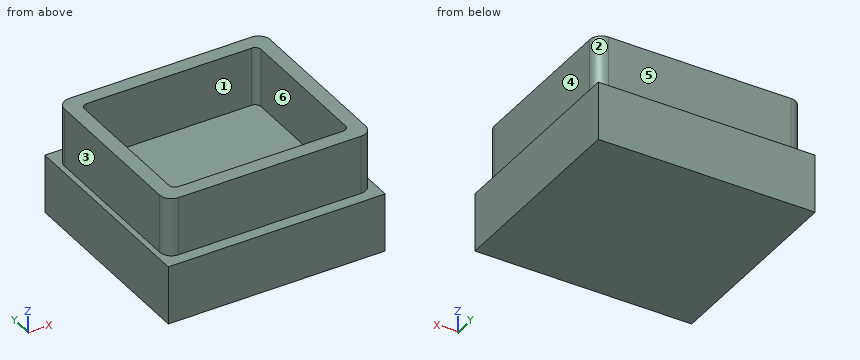
```python
from build123d import *

# Parameters (mm, degrees)
F0_W     = 89.387954
F0_H     = 77.989534
F0_W_2   = 76.687954
F0_H_2   = 65.289534
F1_DEPTH = 25.4
F2_R     = 5.08
F3_R     = 2.54
F4_W     = 94.174876
F4_H     = 87.917894
F5_DEPTH = 25.4


with BuildPart() as f1:
    # F0 (on Top) → F1 (new body)
    with BuildSketch(Plane.XY):
        Rectangle(F0_W, F0_H)
        Rectangle(F0_W_2, F0_H_2, mode=Mode.SUBTRACT)
    extrude(amount=F1_DEPTH)

    # F2
    f2_edges = [f1.edges().sort_by_distance(p)[0] for p in [
        (-44.693977, -38.994767, 12.7),
        (44.693977, -38.994767, 12.7),
        (44.693977, 38.994767, 12.7),
        (-44.693977, 38.994767, 12.7),
    ]]
    fillet(f2_edges, radius=F2_R)

    # F3
    f3_edges = [f1.edges().sort_by_distance(p)[0] for p in [
        (-38.343977, 32.644767, 12.7),
        (38.343977, 32.644767, 12.7),
        (38.343977, -32.644767, 12.7),
        (-38.343977, -32.644767, 12.7),
    ]]
    fillet(f3_edges, radius=F3_R)

    # F4 (on Top) → F5 (join)
    with BuildSketch(Plane.XY):
        Rectangle(F4_W, F4_H)
    extrude(amount=-F5_DEPTH)


solid = f1.part
```
Input: part model. Units: mm. Frame: model coordinates. Face numbers are marked on the shaded views. A direction names the side the tool comes from. Give positions to 0.01 mm unless a question says otherwise; leave off trailing zeros. Loops run counter-clockwise (first coordinate to the right, second up) from the corner with the lowest first, then second, coordinate; pieces in that order, holes last. Notation, with made-up numbers: (-37.75, -32.75) -> (1.25, -32.75) arc R7 ccw to (1.25, -26.75) -> close; hole circle Ø6 at (-37, -27.5). An arc over 180 degrees is marked (long way). Use a Markdown table: item, result.
Q1. First-contact query: P1, Ø20.5, axis at x = -16, z = 12, coming from the +Y side; P2, Ø7.5, axis at x = 13, z = 7, coming from the -Y side; P3, Ø5, axis at x = 16.5, y = 0.5, coming from the +Z side. Flat tips, straight axial feed; report the tip coordinate or a pass-through.
Entries:
| item | result |
|---|---|
| P1 | stops at y = 38.99 |
| P2 | stops at y = -38.99 |
| P3 | stops at z = 0 |
Q2. Ray query, probe 1 along Y at (x, z) = (12, 6.5); probe 2 along X at (y, z) = (-23, 14.5); probe 3 along Z at (x, y) = (18, -29.5). Return the intervals inside material, ascending. Write a range as from..to.
Entries:
| item | result |
|---|---|
| probe 1 | y = -38.99..-32.64, 32.64..38.99 |
| probe 2 | x = -44.69..-38.34, 38.34..44.69 |
| probe 3 | z = -25.4..0 |
Q3. Access query for the marked faces 4, 5 and 6. Directions: +Z, -Z, +X, -X, +Y, -Y. A direction counts if a zero-diameter tool reaches every point of the face in a straight line with its end or side. Return the directions, or none.
Entries:
| item | result |
|---|---|
| face 4 | +Z, +X, +Y, -Y |
| face 5 | +Z, +X, -X, +Y |
| face 6 | +Z |
Q4. Pull-direction query (Y, two-part tool) for the marked faces 1, 2 and 3; classes: pulls with the +Y half, pulls with the -Y half, needs draft (parallel to the pull), parting line crosses it, or undercut.
Entries:
| item | result |
|---|---|
| face 1 | undercut |
| face 2 | pulls with the +Y half |
| face 3 | needs draft |
Q5. Section query C-C, the plane y = 28.5. Return the cut outline in (x, z).
Entries:
| item | result |
|---|---|
| outline | (-47.09, -25.4) -> (47.09, -25.4) -> (47.09, 0) -> (44.69, 0) -> (44.69, 25.4) -> (38.34, 25.4) -> (38.34, 0) -> (-38.34, 0) -> (-38.34, 25.4) -> (-44.69, 25.4) -> (-44.69, 0) -> (-47.09, 0) -> close |
Q6. Section query A-A, the plane z = 17. Return the cut outline in (x, y).
Entries:
| item | result |
|---|---|
| outline | (-44.69, -33.91) arc R5.08 ccw to (-39.61, -38.99) -> (39.61, -38.99) arc R5.08 ccw to (44.69, -33.91) -> (44.69, 33.91) arc R5.08 ccw to (39.61, 38.99) -> (-39.61, 38.99) arc R5.08 ccw to (-44.69, 33.91) -> close; hole (-38.34, -30.1) arc R2.54 ccw to (-35.8, -32.64) -> (35.8, -32.64) arc R2.54 ccw to (38.34, -30.1) -> (38.34, 30.1) arc R2.54 ccw to (35.8, 32.64) -> (-35.8, 32.64) arc R2.54 ccw to (-38.34, 30.1) -> close |
Q7. Section query B-B, the plane x = 31.5. Return the cut outline in (y, z), plus the area to 3 significant figures.
Entries:
| item | result |
|---|---|
| outline | (-43.96, -25.4) -> (43.96, -25.4) -> (43.96, 0) -> (38.99, 0) -> (38.99, 25.4) -> (32.64, 25.4) -> (32.64, 0) -> (-32.64, 0) -> (-32.64, 25.4) -> (-38.99, 25.4) -> (-38.99, 0) -> (-43.96, 0) -> close |
| area | 2,560 mm² |
